```python
from build123d import *

# Parameters (mm, degrees)
ESQUISSE1_W             = 70
ESQUISSE1_H             = 330
BOSS_EXTRU_1_DEPTH      = 6
ESQUISSE2_R             = 2
ESQUISSE2_R_2           = 4
ESQUISSE2_W             = 55
ESQUISSE2_H             = 27.5
ESQUISSE2_W_2           = 50
ESQUISSE2_H_2           = 10
ENL_V_MAT_EXTRU_2_DEPTH = 169.777960647


with BuildPart() as part:
    # Esquisse1 → Boss.-Extru.1 (new body)
    with BuildSketch(Plane.XY):
        Rectangle(ESQUISSE1_W, ESQUISSE1_H)
    extrude(amount=BOSS_EXTRU_1_DEPTH)

    # Esquisse2 → Enlèv. mat.-Extru.2 (cut, through all)
    with BuildSketch(Plane.XY.offset(6)):
        with Locations((-21, 78.5)):
            Circle(ESQUISSE2_R)
        with Locations(Location((21, 78.5, 0), (0, 0, 180))):
            Circle(ESQUISSE2_R)
        with Locations((-22, 135)):
            Circle(ESQUISSE2_R_2)
        with Locations(Location((22, 135, 0), (0, 0, 180))):
            Circle(ESQUISSE2_R_2)
        with Locations(Location((-21, -78.5, 0), (0, 0, 90))):
            Circle(ESQUISSE2_R)
        with Locations(Location((21, -78.5, 0), (0, 0, 270))):
            Circle(ESQUISSE2_R)
        with Locations(Location((-22, -135, 0), (0, 0, 90))):
            Circle(ESQUISSE2_R_2)
        with Locations(Location((22, -135, 0), (0, 0, 270))):
            Circle(ESQUISSE2_R_2)
        with Locations((0, 102.25)):
            Rectangle(ESQUISSE2_W, ESQUISSE2_H)
        with Locations((0, 148)):
            Rectangle(ESQUISSE2_W_2, ESQUISSE2_H_2)
        with Locations((0, -102.25)):
            Rectangle(ESQUISSE2_W, ESQUISSE2_H)
        with Locations((0, -148)):
            Rectangle(ESQUISSE2_W_2, ESQUISSE2_H_2)
    extrude(amount=-ENL_V_MAT_EXTRU_2_DEPTH, mode=Mode.SUBTRACT)


solid = part.part
```
Model file for the job. Use its own axes, mm. A direction names the side the tool comes from. Coordinates: 2 decimals unless noted, no trailing zeros. Write each loop counter-clockwise with the first axis right and the second up, starting at its lowest first coordinate (ties: lowest second). Pieces come first, ordered by that corner, then holes. Notation, with made-up numbers: (-39.75, 13.5) - (17.25, 13.5) arc R34 ccw to (17.25, 45.5) - close; hole circle Ø7 at (66, -8.5). An arc over 180 degrees is marked (long way). One line per question, with ' | ' between items. Start each with the question number.
Q1. Cut at C-C, the plane z = 1.45. Give the number of separate pieces and of enclosed holes in the cut face, then the cut area to 3 significant figures.
Q2. 3-axis set-ups, long thin cutter, end or side, ignore diameter. For faces 5 (the face through (0, 153, 3)), 6 (the face through (0, 165, 3)): which of +Z, -Z, +X, -X, +Y, -Y reach the whole face in a straight line?
Q3. Cut at B-B, the plane x = 11.5. List the corners of the cut face in (y, z), then the cut area to 3 significant figures.
Q4. Pin check, flat tips, straight feed: pin 1 (4.5 mm diameter, centred on x = -21, y = 78.5, fed in from -Z); pin 2 (2.5 mm diameter, centred on x = 21, y = -78.5, fed in from +Z). Stop position of each tip, or through.
Q5. Pull direction X, two halves, no side cores. Call faces 1 (the face through (25, 148, 3)), 2 (the face through (35, -2, 3)), 3 (the face through (22.521, 131.034, 3.042)), 4 (the face through (0, 2, 6)): pulls with the +X half, pulls with the -X half, needs draft (parallel to the pull), parting line crosses it, or undercut.
Q6. Drill centre lines: line 1 (X direction, y = -78.5, z = 4); line 2 (Y direction, x = 0.5, z = 5); line 3 (X direction, y = -135, z = 1.2). Where is each one in solid material? Low to high. Write a range as [from, to].
Q7. Cut at A-A, the plane y = -135. List the corners of the cut face in (x, z), then the cut area to 3 significant figures.
Answer below:
1) separate pieces: 1 | enclosed holes: 12 | area: 18,800 mm^2
2) face 5: +Z, -Z | face 6: +Z, -Z, +X, -X, +Y
3) outline: (-165, 0) - (-153, 0) - (-153, 6) - (-165, 6) - close; (-143, 0) - (-116, 0) - (-116, 6) - (-143, 6) - close; (-88.5, 0) - (88.5, 0) - (88.5, 6) - (-88.5, 6) - close; (116, 0) - (143, 0) - (143, 6) - (116, 6) - close; (153, 0) - (165, 0) - (165, 6) - (153, 6) - close | area: 1,530 mm^2
4) pin 1: z = 0 | pin 2: through
5) face 1: undercut | face 2: pulls with the +X half | face 3: undercut | face 4: needs draft
6) line 1: [-35, -23], [-19, 19], [23, 35] | line 2: [-165, -153], [-143, -116], [-88.5, 88.5], [116, 143], [153, 165] | line 3: [-35, -26], [-18, 18], [26, 35]
7) outline: (-35, 0) - (-26, 0) - (-26, 6) - (-35, 6) - close; (-18, 0) - (18, 0) - (18, 6) - (-18, 6) - close; (26, 0) - (35, 0) - (35, 6) - (26, 6) - close | area: 324 mm^2
